Geometry: final body of the model. Coordinates: model frame, mm. A direction names the side the tool comes from. Give positions to 0.01 mm unless a question says otherwise; leave off trailing zeros. Loops run counter-clockwise (first coordinate to the right, second up) from the corner with the lowest first, then second, coordinate; pieces in that order, holes last. Notation, with made-up numbers: (-22, 49.5) - (8, 49.5) arc R21 cw to (8, 73.5) - close; hole circle Ø6 at (33.25, 3.25). An arc over 180 degrees is marked (long way). Use one line per item in the form item = value.
```python
from build123d import *

# Parameters (mm, degrees)
F0_W     = 24.13
F0_H     = 4
F0_W_2   = 17.78
F1_DEPTH = 5.08
F0_H_2   = 4.35
F2_DEPTH = 50.8
F3_R     = 3.75
F3_W     = 4
F3_H     = 5.08
F4_DEPTH = 101.6
F6_DEPTH = 5.08
F7_R     = 3.75
F7_W     = 4
F7_H     = 5.08
F8_DEPTH = 101.6


with BuildPart() as f1:
    # F0 (on Top) → F1 (new body)
    with BuildSketch(Plane.XY):
        with Locations((38.735, 0)):
            Rectangle(F0_W, F0_H)
        with Locations((17.78, 0)):
            Rectangle(F0_W_2, F0_H)
        Rectangle(F0_W_2, F0_H)
        with Locations((-17.78, 0)):
            Rectangle(F0_W_2, F0_H)
        with Locations((-38.735, 0)):
            Rectangle(F0_W, F0_H)
    extrude(amount=F1_DEPTH)

    # F0 (on Top) → F2 (join)
    with BuildSketch(Plane.XY):
        with Locations((-17.78, -4.175)):
            Rectangle(F0_W_2, F0_H_2)
        with Locations((17.78, -4.175)):
            Rectangle(F0_W_2, F0_H_2)
        with Locations((-17.78, 4.175)):
            Rectangle(F0_W_2, F0_H_2)
        with Locations((17.78, 4.175)):
            Rectangle(F0_W_2, F0_H_2)
    extrude(amount=F2_DEPTH)

    # F3 (on face) → F4 (join)
    with BuildSketch(Plane(origin=(-50.8, 0, 0), x_dir=(0, -1, 0), z_dir=(-1, 0, 0))):
        with Locations((0, 2.54)):
            Circle(F3_R)
        with Locations((0, 2.54)):
            Rectangle(F3_W, F3_H, mode=Mode.SUBTRACT)
    extrude(amount=-F4_DEPTH)

    # F5 (on face) → F6 (join)
    with BuildSketch(Plane.XY.offset(50.8)):
        Polygon((-8.89, -2), (50.8, -2), (50.8, 2), (-50.8, 2), (-50.8, -2), (-26.67, -2), align=None)
    extrude(amount=-F6_DEPTH)

    # F7 (on face) → F8 (join)
    with BuildSketch(Plane(origin=(-50.8, 0, 0), x_dir=(0, -1, 0), z_dir=(-1, 0, 0))):
        with Locations((0, 48.26)):
            Circle(F7_R)
        with Locations((0, 48.26)):
            Rectangle(F7_W, F7_H, mode=Mode.SUBTRACT)
    extrude(amount=-F8_DEPTH)


solid = f1.part
```
(1) Cut plane D-D (x = 23.5). Return the cut outline in (y, z).
Solution:
outline = (-6.35, 0) - (-2.76, 0) arc R3.75 ccw to (2.76, 0) - (6.35, 0) - (6.35, 50.8) - (2.76, 50.8) arc R3.75 ccw to (-2.76, 50.8) - (-6.35, 50.8) - close; hole (-2, 5.71) arc R3.75 cw to (2, 5.71) - (2, 45.09) arc R3.75 cw to (-2, 45.09) - close
(2) Cut plane B-B (z = 23). Return the cut outline in (x, y).
Solution:
outline = (-26.67, -6.35) - (-8.89, -6.35) - (-8.89, -2) - (-26.67, -2) - close; (-26.67, 2) - (-8.89, 2) - (-8.89, 6.35) - (-26.67, 6.35) - close; (8.89, -6.35) - (26.67, -6.35) - (26.67, -2) - (8.89, -2) - close; (8.89, 2) - (26.67, 2) - (26.67, 6.35) - (8.89, 6.35) - close
(3) Material intervals for L1, parallel to X at y = 3.5, z = 24.5; L2, parallel to Y at x = 13, z = 6.5; L3, parallel to Z at x = -21.5, y = -4.25, sorted ascending. Write a range as from..to.
Solution:
L1 = -26.67..-8.89, 8.89..26.67
L2 = -6.35..-2, 2..6.35
L3 = 0..50.8
(4) Access query for faces 4 (the face through (-8.89, -4, 25)), 5 (the face through (18, 5, 50.8)), 6 (the face through (-18, 5, 0)), 7 (the face through (18, -2, 25)), 8 (the face through (-8.89, 4, 25)). Directions: +Z, -Z, +X, -X, +Y, -Y. A direction counts if a zero-diameter tool reaches every point of the face in a straight line with its end or side. Return the directions, or none.
Solution:
face_4 = -Y
face_5 = +Z, +X, -X, +Y
face_6 = -Z, +X, -X, +Y
face_7 = +X, -X
face_8 = +Y
(5) Pin query (flat end, axial travel): P1, Ø1.5, axis at y = 2.5, z = 20.5, coming from the +X side; P2, Ø1.1, axis at x = 16, y = 4.5, coming from the +Z side; P3, Ø4, axis at x = -15, y = 5.5, coming from the -Z side; P4, Ø12, axis at x = -35, z = 18, coming from the -Y side. Return the tip coordinate at first contact, or that it passes through.
Solution:
P1 = 26.67
P2 = 50.8
P3 = 0
P4 = through
(6) Pull-direction query (Z, two-part tool) for faces 1 (the face through (-26.67, 4, 25)), 2 (the face through (50.8, 0, 48)), 3 (the face through (-18, -5, 0)); classes: released by +Z, released by -Z, zero draft, split by the parting line, or undercut.
Solution:
face_1 = undercut
face_2 = zero draft
face_3 = released by -Z
(7) Cut plane A-A (y = 0). Return the cut outline in (x, z).
Solution:
outline = (-50.8, -1.21) - (50.8, -1.21) - (50.8, 6.29) - (-50.8, 6.29) - close; (-50.8, 44.51) - (50.8, 44.51) - (50.8, 52.01) - (-50.8, 52.01) - close
(8) Cut plane C-C (x = 41.5). Return the cut outline in (y, z).
Solution:
outline = circle Ø7.5 at (0, 2.54); circle Ø7.5 at (0, 48.26)
